from build123d import *

# Parameters (mm, degrees)
BOSS_EXTRUDE1_DEPTH = 12.5
BOSS_EXTRUDE2_DEPTH = 1.5
SKETCH3_R           = 2
CUT_EXTRUDE1_DEPTH  = 43.20485754


with BuildPart() as part:
    # Sketch1 → Boss-Extrude1 (new, symmetric)
    with BuildSketch(Plane(origin=(0, 0, 0), x_dir=(0, 0, -1), z_dir=(1, 0, 0))):
        Polygon((0, 0), (-40, 0), (-40, -5), (-5, -5), (-5, -20), (0, -20), align=None)
    extrude(amount=BOSS_EXTRUDE1_DEPTH, both=True)

    # Sketch2 → Boss-Extrude2 (add, symmetric)
    with BuildSketch(Plane(origin=(0, 0, 0), x_dir=(0, 0, -1), z_dir=(1, 0, 0))):
        Polygon((-30, -5), (-5, -20), (-5, -5), align=None)
    extrude(amount=BOSS_EXTRUDE2_DEPTH, both=True)

    # Sketch3 → Cut-Extrude1 (cut, through all)
    with BuildSketch(Plane.XY.offset(5)):
        with Locations((8, -14)):
            Circle(SKETCH3_R)
        with Locations((-8, -14)):
            Circle(SKETCH3_R)
    extrude(amount=-CUT_EXTRUDE1_DEPTH, mode=Mode.SUBTRACT)


solid = part.part
Source: CAD feature listing. Evaluate the final solid. Frame: model axes, mm. A direction names the side the tool comes from. Give positions to 0.01 mm unless a question says otherwise; leave off trailing zeros. Write each loop counter-clockwise with the first axis right and the second up, starting at its lowest first coordinate (ties: lowest second). Pieces come first, ordered by that corner, then holes. Notation, with made-up numbers: M -13,-38.75 L 16,-38.75 A36 cw 16,-1.75 Z; hole C -4.75,-27.75 d6. An arc over 180 degrees is marked long. Return JSON: item names as keys, results as strings. Group by question number.
1) Set-up query: faces 1 (the face through (0, -10, 0)), 2 (the face through (6, -12, 5)), 3 (the face through (-1.5, -9, 12)). Return all of +Z, -Z, +X, -X, +Y, -Y with unobstructed straight access to the full face (end or side cutting, diameter ignored); none if empty.
2) Cut plane B-B, the plane y = -14. Output: boundary loops of the cut face in (x, z), then the cut area to 3 significant figures.
3) Cut plane A-A, the plane x = -8. Output: boundary loops of the cut face in (y, z), then the cut area to 3 significant figures.
4) First-contact query: pin 1 Ø12 at (x, y) = (2, -17.5) entering from +Z; pin 2 Ø5.5 at (x, y) = (-6.5, -15) entering from +Z; pin 3 Ø7.5 at (y, z) = (-14.5, 21) entering from +X. Flat tips, straight axial feed; report the tip coordinate or a pass-through.
5) Draft query along Y for faces 4 (the face through (-12.5, -4.8, 17.1)), 5 (the face through (3, -5, 23)), 6 (the face through (6.526, -12.648, 2.535)). Return one class per face: released by +Y, released by -Y, zero draft, split by the parting line, or undercut.
6) Cut plane D-D, the plane x = 1. Output: boundary loops of the cut face in (y, z), then the cut area to 4 significant figures.
7) Cut plane C-C, the plane z = 23. Output: boundary loops of the cut face in (x, y), then the cut area to 3 significant figures.
8) Ray query, L1, parallel to Y at x = -8, z = 1.95; L2, parallel to Z at x = -6, y = -13.25; L3, parallel to Y at x = -7.25, z = 21.5. Return the intervals inside material, ascending.
Data:
{
 "1": {"face 1": "-Z, +X, -X, +Y, -Y", "face 2": "+Z, +X, -Y", "face 3": "+Z, -X, -Y"},
 "2": {"outline": "M -12.5,0 L -10,0 L -10,5 L -12.5,5 Z; M -6,0 L 6,0 L 6,5 L 1.5,5 L 1.5,15 L -1.5,15 L -1.5,5 L -6,5 Z; M 10,0 L 12.5,0 L 12.5,5 L 10,5 Z", "area": "115 mm²"},
 "3": {"outline": "M -20,0 L -16,0 L -16,5 L -20,5 Z; M -12,0 L 0,0 L 0,40 L -5,40 L -5,5 L -12,5 Z", "area": "255 mm²"},
 "4": {"pin 1": "stops at z = 19.13", "pin 2": "stops at z = 5", "pin 3": "stops at x = 1.5"},
 "5": {"face 4": "zero draft", "face 5": "released by -Y", "face 6": "undercut"},
 "6": {"outline": "M -20,0 L 0,0 L 0,40 L -5,40 L -5,30 L -20,5 Z", "area": "462.5 mm²"},
 "7": {"outline": "M -12.5,-5 L -1.5,-5 L -1.5,-9.2 L 1.5,-9.2 L 1.5,-5 L 12.5,-5 L 12.5,0 L -12.5,0 Z", "area": "138 mm²"},
 "8": {"L1": "y = -20 to -16, -12 to 0", "L2": "z = 0 to 5", "L3": "y = -5 to 0"}
}
